Can you work these out from the model? Positions are in its coordinate system, mm. A direction names the side the tool comes from. Round coordinates to 2 decimals unless told otherwise and drop trailing zeros. Order: outer loops, then holes, each group sorted by start corner. A loop starts at its lowest first (then second) coordinate and runs counter-clockwise, first axis right, second up. Notation, with made-up numbers: (-1.75, 61.5) -> (8.25, 61.5) arc R17 cw to (8.25, 77.5) -> close; hole circle Ø6 at (14.5, 24.5). An arc over 180 degrees is marked (long way). Use a Markdown table: item, result. Add a question column.
Q1. For faces 1 (the face through (3, 0, 13)), 2 (the face through (3, 0, -13)), 3 (the face through (1, -12, 7)), 4 (the face through (3.5, 11.2, -6.6)), 5 (the face through (3.5, 11.2, 6.6)), which set-ups out of +Z, -Z, +X, -X, +Y, -Y let a thin tool reach every point of the face, with its end or its side?
Q2. I'm going to push flat-ended pins straight in: pin 1 Ø3 at (y, z) = (-9, -7) entering from -X; pin 2 Ø3 at (x, z) = (3.5, -2) entering from -Y; pin 3 Ø2.5 at (x, y) = (3, -3) entering from -Z; pin 4 Ø3 at (x, z) = (1.5, 6) entering from -Y. Where does each tip first touch, or does it pass through?
Q3. We'd pull the mould along Z, two halves only. Please class faces 6 (the face through (2.96, -9.03, -2.01)), 7 (the face through (1, -12, -7)), 8 (the face through (3.465, -11.303, -6.422)): +Z half, -Z half, draft (parallel to the pull), parting line (faces both ways), or undercut.
Q4. If we section it at D-D on z = 8.5: List the corners of the cut face in (x, y) for me, plus the area to 3 significant figures.
Q5. If we section it at B-B on x = 3.5: List the corners of the cut face in (y, z) for me.
Q6. If we section it at A-A on z = 0: List the corners of the cut face in (x, y) for me, plus the area to 3 significant figures.
Q7. I need wall thicknesses on line 1 along Y through (x, z) = (2.75, -0.25); line 2 along Z through (x, y) = (3, -6.75); line 3 along Z through (x, y) = (5.75, -3.5). Which ranges of each line are inside material? Lowest first, please. Write a range as [from, to].
Q8. If we section it at C-C on y = 0: List the corners of the cut face in (x, z) for me.
```python
from build123d import *

# Parameters (mm, degrees)
EXTRUDE_1_DEPTH     = 6
SKETCH_3_R          = 14.5
EXTRUDE_2_DEPTH     = 1
SKETCH_4_R          = 15.011106999
SKETCH_4_R_2        = 14.5
CUT_EXTRUDE_1_DEPTH = 22.715969546
SKETCH_5_R          = 9.25
CUT_EXTRUDE_2_DEPTH = 22.365860619


with BuildPart() as part:
    # Эскиз1 → Вытянуть1 (new body)
    with BuildSketch(Plane(origin=(0, 0, 0), x_dir=(0, 0, -1), z_dir=(1, 0, 0))):
        Polygon((0, 15.011106999), (0, -15.011106999), (-13, -7.505553499), (-13, 7.505553499), align=None)
        Polygon((13, 7.505553499), (0, 15.011106999), (0, -15.011106999), (13, -7.505553499), align=None)
    extrude(amount=EXTRUDE_1_DEPTH)

    # Эскиз3 → Вытянуть2 (add)
    with BuildSketch(Plane.ZY):
        Circle(SKETCH_3_R)
    extrude(amount=-EXTRUDE_2_DEPTH)

    # Эскиз4 → Вырез-Вытянуть1 (cut, through all)
    with BuildSketch(Plane.ZY):
        Circle(SKETCH_4_R)
        Circle(SKETCH_4_R_2, mode=Mode.SUBTRACT)
    extrude(amount=-CUT_EXTRUDE_1_DEPTH, mode=Mode.SUBTRACT)

    # Эскиз5 → Вырез-Вытянуть2 (cut, through all)
    with BuildSketch(Plane.ZY):
        Circle(SKETCH_5_R)
    extrude(amount=-CUT_EXTRUDE_2_DEPTH, mode=Mode.SUBTRACT)

    # Эскиз6 → Вырез-Повернуть1 (revolve, cut)
    with BuildSketch(Plane.XY, mode=Mode.PRIVATE) as cut_revolve_1_sk:
        Polygon((4.5, 15.1), (6, 13.6), (6, 15.1), align=None)
    revolve(cut_revolve_1_sk.sketch.rotate(Axis((6, 0, 0), (-1, 0, 0)), 270), axis=Axis((6, 0, 0), (-1, 0, 0)), mode=Mode.SUBTRACT)


solid = part.part
```
Answer below:
| question | item | result |
|---|---|---|
| 1 | face 1 | +Z, +X, +Y, -Y |
| 1 | face 2 | -Z, +X, +Y, -Y |
| 1 | face 3 | +Z, +X, -Y |
| 1 | face 4 | -Z, +X, +Y |
| 1 | face 5 | +Z, +X, +Y |
| 2 | pin 1 | x = 0 |
| 2 | pin 2 | y = -14.49 |
| 2 | pin 3 | z = -13 |
| 2 | pin 4 | y = -13.76 |
| 3 | face 6 | undercut |
| 3 | face 7 | draft |
| 3 | face 8 | -Z half |
| 4 | outline | (0, -11.75) -> (1, -11.75) -> (1, -10.1) -> (6, -10.1) -> (6, -3.65) -> (0, -3.65) -> close; (0, 3.65) -> (6, 3.65) -> (6, 10.1) -> (1, 10.1) -> (1, 11.75) -> (0, 11.75) -> close |
| 4 | area | 80.7 mm² |
| 5 | outline | (-14.47, -0.94) -> (-8.05, -12.06) arc R14.5 ccw to (-6.42, -13) -> (6.42, -13) arc R14.5 ccw to (8.05, -12.06) -> (14.47, -0.94) arc R14.5 ccw to (14.47, 0.94) -> (8.05, 12.06) arc R14.5 ccw to (6.42, 13) -> (-6.42, 13) arc R14.5 ccw to (-8.05, 12.06) -> (-14.47, 0.94) arc R14.5 ccw to start; hole circle Ø18.5 at (0, 0) |
| 6 | outline | (0, -14.5) -> (5.1, -14.5) -> (6, -13.6) -> (6, -9.25) -> (0, -9.25) -> close; (0, 9.25) -> (6, 9.25) -> (6, 13.6) -> (5.1, 14.5) -> (0, 14.5) -> close |
| 6 | area | 62.2 mm² |
| 7 | line 1 | [-14.5, -9.25], [9.25, 14.5] |
| 7 | line 2 | [-12.83, -6.32], [6.32, 12.83] |
| 7 | line 3 | [-13, -8.56], [8.56, 13] |
| 8 | outline | (0, -14.5) -> (1, -14.5) -> (1, -13) -> (6, -13) -> (6, -9.25) -> (0, -9.25) -> close; (0, 9.25) -> (6, 9.25) -> (6, 13) -> (1, 13) -> (1, 14.5) -> (0, 14.5) -> close |
